```python
from build123d import *
from build123d import SkipClean  # not in build123d's __all__

# Parameters (mm, degrees)
F0_R     = 45
F1_DEPTH = 5
F2_R     = 2.5
F3_DEPTH = 65
F7_DEPTH = 5.0010001144


# Not quite as in the source:
# - a feature of the source that left no trace in its solid (it failed there, or was rolled back) is left out
# - a feature names something its author has since deleted; it is built from what else it names


with BuildPart() as f1:
    # F0 (on Front) → F1 (new body)
    with BuildSketch(Plane.XZ):
        Circle(F0_R)
    extrude(amount=F1_DEPTH)

    # F2 (on Top) → F3 (join)
    with BuildSketch(Plane.XY):
        with Locations((0, -2.5)):
            Circle(F2_R)
    with SkipClean():  # cleaning this boolean's faces spoils the solid; the shape is the same uncleaned
        extrude(amount=-F3_DEPTH)

    # F6 (on face) → F7 (cut, through all)
    with BuildSketch(Plane.XZ.offset(5)):
        Polygon((-20.7163122443, 7.7645383693), (-18, 17), (-38, 17), (-35.2836877557, 7.7645383693), align=None)
        with BuildLine():
            Line((-36.1941438848, -2.7399107917), (-40.3882877696, 11.5201784167))
            ThreePointArc((-40.3882877696, 11.5201784167), (-41.3363102402, 4.4204212554), (-41.1493788917, -2.7399107917))
            Line((-41.1493788917, -2.7399107917), (-36.1941438848, -2.7399107917))
        make_face()
        with BuildLine():
            Line((-32, -17), (-35.2739794285, -5.8684699433))
            Line((-35.2739794285, -5.8684699433), (-40.7068101942, -5.8684699433))
            ThreePointArc((-40.7068101942, -5.8684699433), (-39.3148104816, -11.548035888), (-37.2002845672, -17))
            Line((-37.2002845672, -17), (-32, -17))
        make_face()
        Polygon((-24.4349641852, -4.8788782297), (-21.5628112163, 4.8864418646), (-34.4371887837, 4.8864418646), (-31.5650358148, -4.8788782297), align=None)
        Polygon((-28, -17), (-25.2814631572, -7.7569747344), (-30.7185368428, -7.7569747344), align=None)
        Polygon((-11.2836877557, 7.7645383693), (-14, 17), (-16.7163122443, 7.7645383693), align=None)
        Polygon((-7.5650358148, -4.8788782297), (-10.4371887837, 4.8864418646), (-17.5628112163, 4.8864418646), (-20.4349641852, -4.8788782297), align=None)
        Polygon((-4, -17), (-6.7185368428, -7.7569747344), (-21.2814631572, -7.7569747344), (-24, -17), align=None)
        Polygon((0, -7.7569747344), (-2.7185368428, -7.7569747344), (0, -17), align=None)
        Polygon((0, -7.7569747344), (0, -17), (2.7185368428, -7.7569747344), align=None)
        Polygon((6.4371887837, 4.8864418646), (0, 4.8864418646), (0, 0), (0, -4.8788782297), (3.5650358148, -4.8788782297), align=None)
        Polygon((0, 4.8864418646), (-6.4371887837, 4.8864418646), (-3.5650358148, -4.8788782297), (0, -4.8788782297), (0, 0), align=None)
        Polygon((0, 17), (-10, 17), (-7.2836877557, 7.7645383693), (0, 7.7645383693), align=None)
        Polygon((10, 17), (0, 17), (0, 7.7645383693), (7.2836877557, 7.7645383693), align=None)
        Polygon((16.7163122443, 7.7645383693), (14, 17), (11.2836877557, 7.7645383693), align=None)
        Polygon((17.5628112163, 4.8864418646), (10.4371887837, 4.8864418646), (7.5650358148, -4.8788782297), (20.4349641852, -4.8788782297), align=None)
        Polygon((21.2814631572, -7.7569747344), (6.7185368428, -7.7569747344), (4, -17), (24, -17), align=None)
        Polygon((25.2814631572, -7.7569747344), (28, -17), (30.7185368428, -7.7569747344), align=None)
        Polygon((24.4349641852, -4.8788782297), (31.5650358148, -4.8788782297), (34.4371887837, 4.8864418646), (21.5628112163, 4.8864418646), align=None)
        Polygon((20.7163122443, 7.7645383693), (35.2836877557, 7.7645383693), (38, 17), (18, 17), align=None)
        with BuildLine():
            ThreePointArc((41.1493788917, -2.7399107917), (41.3363102402, 4.4204212554), (40.3882877696, 11.5201784167))
            Line((40.3882877696, 11.5201784167), (36.1941438848, -2.7399107917))
            Line((36.1941438848, -2.7399107917), (41.1493788917, -2.7399107917))
        make_face()
        with BuildLine():
            Line((40.7068101942, -5.8684699433), (35.2739794285, -5.8684699433))
            Line((35.2739794285, -5.8684699433), (32, -17))
            Line((32, -17), (37.2002845672, -17))
            ThreePointArc((37.2002845672, -17), (39.3148104816, -11.548035888), (40.7068101942, -5.8684699433))
        make_face()
    with SkipClean():  # cleaning this boolean's faces spoils the solid; the shape is the same uncleaned
        extrude(amount=-F7_DEPTH, mode=Mode.SUBTRACT)


solid = f1.part
```
Design review of the part built by this model. Coordinates are the model's own, in mm. Coordinates: 2 decimals unless noted, no trailing zeros. Order: outer loops, then holes, each group sorted by start corner. A loop starts at its lowest first (then second) coordinate and runs counter-clockwise, first axis right, second up.
1) Take a section at A-A, the plane y = -2.5. State how many separate pieces and enclosed holes the cut face has, and give its area (3 significant figures).
2) Take a section at B-B, the plane z = -49. Give the boundary of the cut face in (x, y).
3) Wall thickness on line 1 along X through (y, z) = (-4.2, -6); line 2 along Z through (x, y) = (-25, -4.55); line 3 along Z through (x, y) = (7, -3.9): over which ranges is each line inside the solid? List them lowest first.
4) Take a section at C-C, the plane z = 37. Give the boundary of the cut face in (x, y).
5) Take a section at D-D, the plane z = -18.5. Give the boundary of the cut face in (x, y).
6) Clearance check with flat-ended pins moving along their axes: pin 1 (2.5 mm diameter, centred on x = -12, y = -2, fed in from +Z); pin 2 (2.5 mm diameter, centred on x = -27.5, y = -3, fed in from +Z); pin 3 (2 mm diameter, centred on x = -24.5, y = -4.5, fed in from +Z). State where each tip first meets the part, or that it passes through.
Returned:
1. separate pieces: 1
1. enclosed holes: 19
1. area: 4,840 mm2
2. outline: circle Ø5 at (0, -2.5)
3. line 1: x = -44.6 to -40.68, -35.24 to 35.24, 40.68 to 44.6
3. line 2: z = -37.42 to -4.88, 4.89 to 7.76, 17 to 37.42
3. line 3: z = -44.45 to -17, -7.76 to 7.76, 17 to 44.45
4. outline: (-25.61, -5) - (25.61, -5) - (25.61, 0) - (-25.61, 0) - close
5. outline: (-41.02, -5) - (41.02, -5) - (41.02, 0) - (-41.02, 0) - close
6. pin 1: stops at z = 43.7
6. pin 2: stops at z = 36.55
6. pin 3: stops at z = 38.38
